Autodesk Inventor part; units mm, degrees
ref_plane "YZ Plane" through (0, 0, 0) normal (1, 0, 0) x (0, 1, 0)
ref_plane "XZ Plane" through (0, 0, 0) normal (0, 1, 0) x (-1, 0, 0)
ref_plane "XY Plane" through (0, 0, 0) normal (0, 0, 1) x (1, 0, 0)
sketch "Sketch1" plane through (0, 0, 0) normal (0, 1, 0) x (-1, 0, 0)
  line L0 (0, 0) -> (7, 0)
  line L1 (7, 0) -> (7, -6.684)
  line L2 (7, -6.684) -> (0, -6.684)
  line L3 (0, -6.684) -> (0, 0)
  line L4 (3.5, -6.684) -> (3.5, -3.342)
  circle A0 centre (3.5, -3.342) radius 1.75
  dimension "d0" = 7
  dimension "d1" = 6.684
  dimension "d2" = 3.342
  dimension "d3" = 3.5
extrude "Extrusion1" add sketch "Sketch1" along normal blind 1
sketch "Sketch2" plane through (0, 1, 0) normal (0, 1, 0) x (1, 0, 0)
  line L0 (-7, 6.684) -> (-7, 0)
  line L1 (-7, 0) -> (0, 0)
  line L2 (0, 0) -> (0, 6.684)
  line L3 (0, 6.684) -> (-7, 6.684)
  circle A0 centre (-3.5, 3.342) radius 1.75
  arc A1 (-7, 0) -> (0, 0) centre (-3.5, 0) ccw
extrude "Extrusion2" add sketch "Sketch2" along normal blind 1
properties part number "sunfoundernub"
Input: part model. Units: mm. Frame: model coordinates. A direction names the side the tool comes from. Give positions to 0.01 mm unless a question says otherwise; leave off trailing zeros. Write each loop counter-clockwise with the first axis right and the second up, starting at its lowest first coordinate (ties: lowest second). Pieces come first, ordered by that corner, then holes. Notation, with made-up numbers: (84.5, 83) - (103.5, 83) arc R23 cw to (103.5, 113) - close; hole circle Ø4 at (50.5, 13.25). An arc over 180 degrees is marked (long way). Write item = value, one per line. Start each with the question number.
1. Mould query, pull axis X, two halves, no side actions, for faces 3 (the flat face through (-4, 1, -6.684)), 4 (the cylindrical face through (-3.4, 1.5, 3.5)), 5 (the cylindrical face through (-3.385, 1.208, -1.596)). Classes: released by +X, released by -X, zero draft, split by the parting line, or undercut.
2. Section query A-A, the plane z = -3.5. Output: boundary loops of the cut face in (x, y).
3. Section query B-B, the plane y = 1.65. Output: boundary loops of the cut face in (x, z), then the cut area to 3 significant figures.
4. Access query for faces 1 (the flat face through (-3.5, 0.5, 0)), 2 (the flat face through (0, 1, -3)). Directions: +Z, -Z, +X, -X, +Y, -Y. A direction counts if a zero-diameter tool reaches every point of the face in a straight line with its end or side. Return the directions, or none.
5. Section query D-D, the plane y = 0.4. Output: boundary loops of the cut face in (x, z).
6. Ray query, L1, parallel to Z at x = -3.5, y = 0.95; L2, parallel to Z at x = -3.5, y = 1.4; L3, parallel to X at y = 1.45, z = -2.25. Return the intervals inside material, ascending.
7. First-contact query: pin 1 Ø1 at (x, z) = (-2, 2) entering from -Y; pin 2 Ø1 at (x, z) = (-4, -3) entering from +Y. Flat tips, straight axial feed; report the tip coordinate or a pass-through.
Check sheet entries:
q1.face_3 = zero draft
q1.face_4 = split by the parting line
q1.face_5 = undercut
q2.outline = (-7, 0) - (-5.24, 0) - (-5.24, 2) - (-7, 2) - close; (-1.76, 0) - (0, 0) - (0, 2) - (-1.76, 2) - close
q3.outline = (-7, -6.68) - (0, -6.68) - (0, 0) arc R3.5 ccw to (-7, 0) - close; hole circle Ø3.5 at (-3.5, -3.34)
q3.area = 56.4 mm2
q4.face_1 = +Z, +X, -X, -Y
q4.face_2 = +Z, -Z, +X, +Y, -Y
q5.outline = (-7, -6.68) - (0, -6.68) - (0, 0) - (-7, 0) - close; hole circle Ø3.5 at (-3.5, -3.34)
q6.L1 = -6.68 to -5.09, -1.59 to 0
q6.L2 = -6.68 to -5.09, -1.59 to 3.5
q6.L3 = -7 to -4.87, -2.13 to 0
q7.pin_1 = 1
q7.pin_2 = through
